Source: three-view drawing plus pictorial views. Frame: mm from the lowest corner of the part. A direction names the side the tool comes from. Give positions to 0.01 mm unless a question says otherwise; leave off trailing zeros. Write each loop counter-clockwise with the first axis right and the second up, starting at its lowest first coordinate (ties: lowest second). Pieces come first, ordered by that corner, then holes. Notation, with made-up numbers: (-33.75, -25.5) -> (-24.75, -25.5) arc R28 ccw to (-24.75, 8.5) -> close; hole circle Ø8 at (74.5, -23.75). An arc over 180 degrees is marked (long way). Write item = value, one per line.
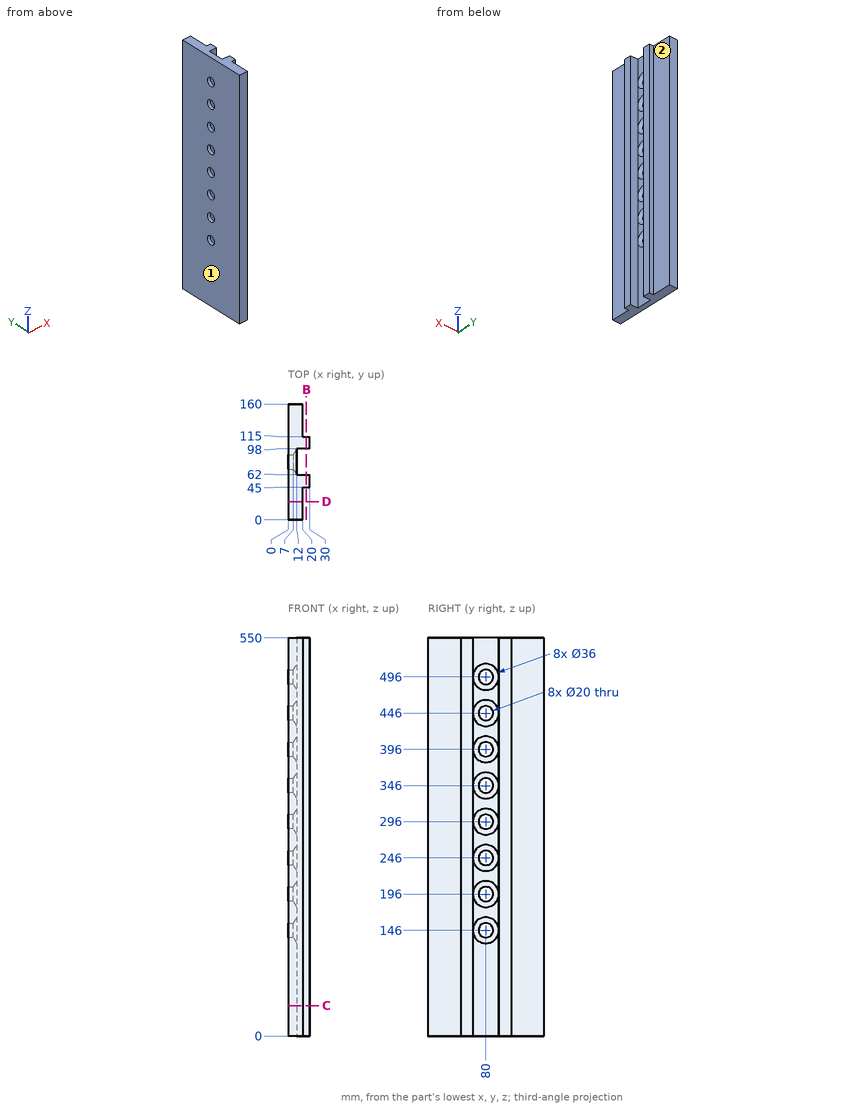
1) Cut plane B-B (x = 25). Return the cut outline in (y, z).
Computed:
outline = (45, 0) -> (62, 0) -> (62, 550) -> (45, 550) -> close; (98, 0) -> (115, 0) -> (115, 550) -> (98, 550) -> close
2) Cut plane C-C (z = 42). Return the cut outline in (x, y), then the cut area to 3 significant figures.
Computed:
outline = (0, 0) -> (20, 0) -> (20, 45) -> (30, 45) -> (30, 62) -> (12, 62) -> (12, 98) -> (30, 98) -> (30, 115) -> (20, 115) -> (20, 160) -> (0, 160) -> close
area = 3,250 mm²
3) Access query for the marked faces 1 and 2. Directions: +Z, -Z, +X, -X, +Y, -Y. A direction counts if a zero-diameter tool reaches every point of the face in a straight line with its end or side. Return the directions, or none.
Computed:
face_1 = +Z, -Z, -X, +Y, -Y
face_2 = +Z, -Z, +X, +Y
4) Cut plane D-D (y = 25). Return the cut outline in (x, z), then the cut area to 3 significant figures.
Computed:
outline = (0, 0) -> (20, 0) -> (20, 550) -> (0, 550) -> close
area = 11,000 mm²
5) Contact query for flat-ended pins moving along their axis: pin 1 (3 mm diameter, centred on x = 25.5, z = 253.5, fed in from +Y); pin 2 (22.5 mm diameter, centred on y = 21.5, z = 259.5, fed in from +X). Output: stop coordinate, or through.
Computed:
pin_1 = 115
pin_2 = 20
6) Material intervals for L1, parallel to Y at x = 12.75, z = 496.5; L2, parallel to Y at x = 3, z = 196; L3, parallel to X at y = 19.5, z = 33.5, sorted ascending.
Computed:
L1 = 0 to 62, 98 to 160
L2 = 0 to 70, 90 to 160
L3 = 0 to 20
